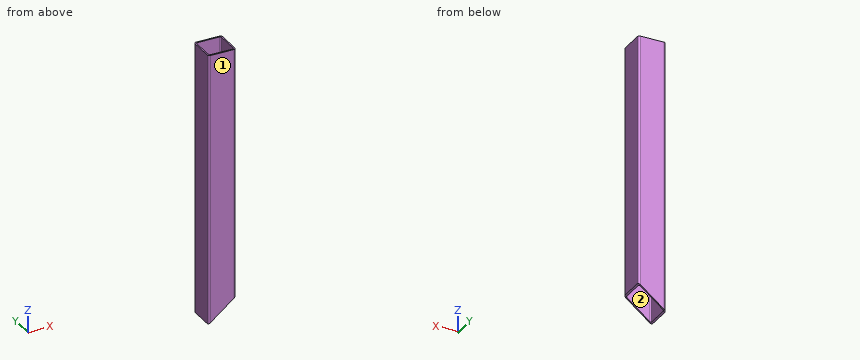
Autodesk Inventor part; units mm, degrees
ref_plane "Start Plane" through (0, 0, 24.1171) normal (0, 0, 1) x (1, 0, 0)
ref_plane "End Plane" through (0, 0, 1009.5) normal (0, 0, 1) x (1, 0, 0)
ref_plane "Work Plane6" through (460.6876, 42.5, 430.3364) normal (0.6225, 0, -0.7826) x (-0.7826, 0, -0.6225)
ref_plane "Start Plane" through (0, 0, 24.1171) normal (0, 0, 1) x (1, 0, 0)
ref_plane "End Plane" through (0, 0, 1009.5) normal (0, 0, 1) x (1, 0, 0)
sketch "Sketch" plane through (0, 0, 0) normal (0, 0, 1) x (1, 0, 0)
  line L0 (-50, -42.5) -> (-50, 42.5)
  line L1 (-42.5, 50) -> (42.5, 50)
  line L2 (50, 42.5) -> (50, -42.5)
  line L3 (42.5, -50) -> (-42.5, -50)
  arc A0 (-50, -42.5) -> (-42.5, -50) centre (-42.5, -42.5) ccw
  arc A1 (-42.5, 50) -> (-50, 42.5) centre (-42.5, 42.5) ccw
  arc A2 (50, 42.5) -> (42.5, 50) centre (42.5, 42.5) ccw
  arc A3 (42.5, -50) -> (50, -42.5) centre (42.5, -42.5) ccw
  line L4 (-40, 45) -> (40, 45)
  line L5 (45, 40) -> (45, -40)
  line L6 (40, -45) -> (-40, -45)
  line L7 (-45, -40) -> (-45, 40)
  line L8 (0, 72.1746) -> (0, -72.1746) construction
  line L9 (-72.1746, 0) -> (72.1746, 0) construction
  arc A4 (-45, -40) -> (-40, -45) centre (-40, -40) ccw
  arc A5 (-40, 45) -> (-45, 40) centre (-40, 40) ccw
  arc A6 (45, 40) -> (40, 45) centre (40, 40) ccw
  arc A7 (40, -45) -> (45, -40) centre (40, -40) ccw
  dimension "d7" = 7.5
  dimension "d10" = 100
  dimension "d11" = 100
  dimension "d12" = 5
  dimension "d15" = 50
  dimension "d16" = 50
  dimension "d19" = 5
  dimension "d20" = 5
extrude "Body" add sketch "Sketch" along normal up to surface (985.3829 mm away) from surface at 24.1171
sketch "Sketch3" plane through (0, 0, 0) normal (0, 0, 1) x (1, 0, 0)
  line L0 (0, 0) -> (10, 0)
ref_plane "Work Plane3" through (0, 0, 0) normal (0, -1, 0) x (1, 0, 0)
ref_plane "Work Plane6" through (460.6876, 42.5, 430.3364) normal (0.6225, 0, -0.7826) x (-0.7826, 0, -0.6225)
split "Split3" plane through (460.6876, 42.5, 430.3364) removes the side toward (0.6225, 0, -0.7826)
sketch "Sketch4" plane through (0, 0, 0) normal (0, -1, 0) x (1, 0, 0)
  line L0 (-2, 24.1171) -> (12, 24.1171)
  line L1 (-2, 1009.5) -> (12, 1009.5)
  dimension "d18" = 985.3829
equation "\"d7\" = G_IR"
equation "\"d10\" = G_H"
equation "\"d11\" = G_W"
equation "\"d12\" = G_T"
equation "\"d15\" = 0.5 * d10"
equation "\"d16\" = 0.5 * d11"
equation "\"d19\" = G_T"
equation "\"d20\" = G_T"
equation "\"d3\" = G_L"
equation "\"G_W\" = 100"
equation "\"G_H\" = 100"
equation "\"G_T\" = 5"
equation "\"G_IR\" = 7.5"
equation "\"G_L\" = d18"
equation "\"G_OFFSET_START\" = -24.11714"
equation "\"G_OFFSET_END\" = 0"
equation "\"d13\" = -G_OFFSET_START"
equation "\"d14\" = G_OFFSET_END + B_L"
equation "\"B_L\" = 1009.5"
properties part number "DIN EN 10210-2 - 100 x 100 x 5 - 985,38" material "Steel, Mild"
Design review of the part built by this model. Coordinates are the model's own, in mm. Face numbers are marked on the shaded views. A direction names the side the tool comes from. Round coordinates to 2 decimals unless told otherwise and drop trailing zeros. Write each loop counter-clockwise with the first axis right and the second up, starting at its lowest first coordinate (ties: lowest second). Pieces come first, ordered by that corner, then holes. Notation, with made-up numbers: (0.5, 30) - (17.5, 30) arc R26 cw to (17.5, 51) - close; hole circle Ø8 at (8, 30). An arc over 180 degrees is marked (long way). Return JSON: item names as keys, results as strings. Group by question number.
Item 1: Machinability: for the marked faces 1 and 2, which of the approach directions +Z, -Z, +X, -X, +Y, -Y give a long, thin tool a straight path to every point of the face, cutting with its end or side? Answer none if there is none.
Item 2: For probe 1 along X at (y, z) = (17.5, 405); probe 2 along X at (y, z) = (-41, 276.5), list the stretches that pass through material, from the lowest coordinate up. Write a range as [from, to].
Item 3: We need section A-A on y = -24.5. Write out the cut boundary in (x, z), and give its area (3 significant figures).
Item 4: We need section C-C on x = 24. Write out the cut boundary in (y, z).
Item 5: We need section B-B on z = 678.5. Write out the cut boundary in (x, y).
Model answer:
{
 "1": {"face 1": "+Z, -Z, +X, -X, -Y", "face 2": "+Z, -Z"},
 "2": {"probe 1": "x = [-50, -45], [45, 50]", "probe 2": "x = [-50, -44.9], [44.9, 50]"},
 "3": {"outline": "(-50, 24.12) - (-45, 28.09) - (-45, 1009.5) - (-50, 1009.5) - close; (45, 99.68) - (50, 103.66) - (50, 1009.5) - (45, 1009.5) - close", "area": "9,460 mm²"},
 "4": {"outline": "(-50, 82.98) - (-45, 82.98) - (-45, 1009.5) - (-50, 1009.5) - close; (45, 82.98) - (50, 82.98) - (50, 1009.5) - (45, 1009.5) - close"},
 "5": {"outline": "(-50, -42.5) arc R7.5 ccw to (-42.5, -50) - (42.5, -50) arc R7.5 ccw to (50, -42.5) - (50, 42.5) arc R7.5 ccw to (42.5, 50) - (-42.5, 50) arc R7.5 ccw to (-50, 42.5) - close; hole (-45, -40) arc R5 ccw to (-40, -45) - (40, -45) arc R5 ccw to (45, -40) - (45, 40) arc R5 ccw to (40, 45) - (-40, 45) arc R5 ccw to (-45, 40) - close"}
}
